Verification items for the finished model (mm, model axes). A direction names the side the tool comes from. Coordinates: 2 decimals unless noted, no trailing zeros. Order: outer loops, then holes, each group sorted by start corner. A loop starts at its lowest first (then second) coordinate and runs counter-clockwise, first axis right, second up. Notation, with made-up numbers: (-17, 26) -> (20, 26) arc R8 cw to (20, 41) -> close; hole circle Ø7 at (46, -8.5). An arc over 180 degrees is marked (long way). Use CSV: the item, a comma, the result in double quotes. Start each with the question number.
1) Tool access check on faces 1 (the flat face through (14, 0, 5)), 2 (the flat face through (15, 13.716, 19)), 3 (the flat face through (36.906, 13, 15)). Record the directions out of +Z, -Z, +X, -X, +Y, -Y that give a thin tool (end or side, any length) a straight path to the whole face; none if there is none.
2) Sectioned sample at C-C on y = 1. Record the boundary of the cut face in (x, z).
3) Release check for a two-part mould opening along Z. For faces 4 (the flat face through (14, -2, 11.112)), 5 (the cylindrical face through (27.86, 17.47, 31.99)), 6 (the cylindrical face through (-5.36, -5.23, 5.63)) record: released by +Z, released by -Z, zero draft, split by the parting line, or undercut.
4) Sectioned sample at A-A on x = 8. Record the boundary of the cut face in (y, z), then the cut area to 3 significant figures.
5) Sectioned sample at B-B on z = 8.5. Record the boundary of the cut face in (x, y) (1 decimal).
6) Go/stop test with flat-tipped pins: pin 1 (4 mm diameter, centred on x = 8, y = -3.5, fed in from +Z); pin 2 (8 mm diameter, centred on y = 6.5, z = 28.5, fed in from -X). Record where each tip stops, or that it passes through.
7) Scan lines: line 1 along X through (y, z) = (9, 4.5); line 2 along Y through (x, z) = (8, 2); line 3 along X through (y, z) = (14.75, 31). Record each from-to range of solid material in increasing order.
8) Sectioned sample at D-D on z = 33. Record the boundary of the cut face in (x, y).
Autodesk Inventor part; units mm, degrees
ref_plane "YZ Plane" through (0, 0, 0) normal (1, 0, 0) x (0, 1, 0)
ref_plane "XZ Plane" through (0, 0, 0) normal (0, 1, 0) x (-1, 0, 0)
ref_plane "XY Plane" through (0, 0, 0) normal (0, 0, 1) x (1, 0, 0)
sketch "Sketch1" plane through (0, 0, 0) normal (0, 0, 1) x (1, 0, 0)
  line L0 (0, 0) -> (29.2862, 0)
  line L1 (29.2862, 0) -> (29.2862, 13.716)
  line L2 (29.2862, 13.716) -> (0, 13.716)
  line L3 (0, 13.716) -> (0, 0)
  line L4 (14.6431, 13.716) -> (14.6431, 0) construction
  line L5 (0, 6.858) -> (29.2862, 6.858) construction
  line L6 (-7.62, -7.62) -> (36.9062, -7.62)
  line L7 (36.9062, -7.62) -> (36.9062, 21.336)
  line L8 (36.9062, 21.336) -> (-7.62, 21.336)
  line L9 (-7.62, 21.336) -> (-7.62, -7.62)
  line L10 (-7.62, -7.62) -> (36.9062, 21.336) construction
  line L11 (36.9062, -7.62) -> (-7.62, 21.336) construction
  point P0 (14.6431, 6.858)
  dimension "d0" = 29.2862
  dimension "d1" = 13.716
  dimension "d2" = 7.62
  dimension "d3" = 7.62
extrude "Extrusion1" add sketch "Sketch1" along normal blind 11.1125
sketch "Sketch2" plane through (0, 0, 11.1125) normal (0, 0, 1) x (1, 0, 0)
  line L0 (0, 13.716) -> (29.2862, 13.716)
  line L1 (36.9062, -7.62) -> (36.9062, 21.336)
  line L2 (36.9062, 21.336) -> (-7.62, 21.336)
  line L3 (-7.62, 21.336) -> (-7.62, -7.62)
  line L4 (-7.62, 13.716) -> (0, 13.716)
  line L5 (29.2862, 13.716) -> (36.9062, 13.716)
extrude "Extrusion2" add sketch "Sketch2" along normal blind 26.9875
sketch "Sketch3" plane through (0, 13.716, 0) normal (0, -1, 0) x (1, 0, 0)
  line L0 (36.9062, 11.1125) -> (36.9062, 38.1)
  line L1 (-7.62, 11.1125) -> (-7.62, 38.1)
  line L2 (-7.62, 31.837) -> (36.9062, 31.837) construction
  circle A0 centre (-2.1601, 31.837) radius 3.5719
  circle A1 centre (31.4297, 31.837) radius 3.5719
  dimension "d8" = 7.1437
  dimension "d9" = 7.1437
extrude "Extrusion3" cut sketch "Sketch3" against normal through all
fillet "Fillet1" radius 7.9375 2 edges at (33.0962, 13.716, 11.1125) (-3.81, 13.716, 11.1125)
fillet "Fillet2" radius 7.9375 2 edges at (-7.62, -7.62, 5.5563) (36.9062, -7.62, 5.5563)
properties part number "switch Holder"
Answers follow:
1,face 1,"+Z, -Z"
1,face 2,"+Z"
1,face 3,"+Z, -Z, +X, +Y, -Y"
2,outline,"(-7.62, 0) -> (0, 0) -> (0, 11.11) -> (-7.62, 11.11) -> close; (29.29, 0) -> (36.91, 0) -> (36.91, 11.11) -> (29.29, 11.11) -> close"
3,face 4,"released by +Z"
3,face 5,"undercut"
3,face 6,"zero draft"
4,outline,"(-7.62, 0) -> (0, 0) -> (0, 11.11) -> (-7.62, 11.11) -> close; (13.72, 0) -> (21.34, 0) -> (21.34, 38.1) -> (13.72, 38.1) -> close"
4,area,"375 mm²"
5,outline,"(-7.6, 0.3) arc R7.9 ccw to (0.3, -7.6) -> (29, -7.6) arc R7.9 ccw to (36.9, 0.3) -> (36.9, 21.3) -> (-7.6, 21.3) -> close; hole (0, 0) -> (29.3, 0) -> (29.3, 13.7) -> (0, 13.7) -> close"
6,pin 1,"stops at z = 11.11"
6,pin 2,"passes through"
7,line 1,"x = -7.62 to 0, 29.29 to 36.91"
7,line 2,"y = -7.62 to 0, 13.72 to 21.34"
7,line 3,"x = -7.62 to -5.63, 1.31 to 27.96, 34.9 to 36.91"
8,outline,"(-7.62, 13.72) -> (-5.54, 13.72) -> (-5.54, 21.34) -> (-7.62, 21.34) -> close; (1.22, 13.72) -> (28.05, 13.72) -> (28.05, 21.34) -> (1.22, 21.34) -> close; (34.81, 13.72) -> (36.91, 13.72) -> (36.91, 21.34) -> (34.81, 21.34) -> close"
